Design review of the part built by this model. Coordinates are the model's own, in mm. A direction names the side the tool comes from. Coordinates: 2 decimals unless noted, no trailing zeros. Loops run counter-clockwise (first coordinate to the right, second up) from the corner with the lowest first, then second, coordinate; pieces in that order, holes last. Notation, with made-up numbers: (-17, 27) -> (36, 27) arc R12 cw to (36, 46) -> close; hole circle Ø10 at (-0.5, -10.5). An arc over 180 degrees is marked (long way). Answer in a Markdown table with one row per item.
```python
from build123d import *

# Parameters (mm, degrees)
SKETCH_1_R          = 7.25
SKETCH_1_R_2        = 4
EXTRUDE_1_DEPTH     = 6
SKETCH_2_R          = 3
SKETCH_2_R_2        = 1.5
CUT_EXTRUDE_1_DEPTH = 6


with BuildPart() as part:
    # 草图1 → 凸台-拉伸1 (new body)
    with BuildSketch(Plane.XY):
        with Locations((-10.375, 0)):
            Circle(SKETCH_1_R)
        with BuildLine():
            ThreePointArc((13.625, -4), (9.625, 0), (13.625, 4))
            Line((13.625, 4), (-4.328306689, 4))
            ThreePointArc((-4.328306689, 4), (-3.432341053, 2.088536987), (-3.125, 0))
            ThreePointArc((-3.125, 0), (-3.432341053, -2.088536987), (-4.328306689, -4))
            Line((-4.328306689, -4), (13.625, -4))
        make_face()
        with Locations((13.625, 0)):
            Circle(SKETCH_1_R_2)
    extrude(amount=EXTRUDE_1_DEPTH)

    # 草图2 → 切除-拉伸1 (cut)
    with BuildSketch(Plane.XY.offset(6)):
        with Locations((-10.375, 0)):
            Circle(SKETCH_2_R)
        with Locations((13.625, 0)):
            Circle(SKETCH_2_R_2)
    extrude(amount=-CUT_EXTRUDE_1_DEPTH, mode=Mode.SUBTRACT)


solid = part.part
```
(1) For pin 1 (2 mm diameter, centred on y = 4, z = 1, fed in from +X); pin 2 (6 mm diameter, centred on x = 5, y = 2, fed in from -Z); pin 3 (1 mm diameter, centred on x = -13, z = 3.5, fed in from +Y); pin 4 (2.5 mm diameter, centred on x = 13.625, y = 0, fed in from -Z), all flat-tipped, find the tip position at first contact; note any pin that passes through.
Evaluation:
| item | result |
|---|---|
| pin 1 | stops at x = 16.27 |
| pin 2 | stops at z = 0 |
| pin 3 | stops at y = 6.93 |
| pin 4 | passes through |
(2) Take a section at D-D on x = 2.5. Give the boundary of the cut face in (y, z).
Evaluation:
| item | result |
|---|---|
| outline | (-4, 0) -> (4, 0) -> (4, 6) -> (-4, 6) -> close |
(3) To check wall thickness, follow probe 1 along X at (y, z) = (-0.25, 2.2); probe 2 along Y at (x, z) = (-10.5, 0.7); probe 3 along Y at (x, z) = (-9.5, 5.45). State the ranges of each line that lie inside material, in increasing order.
Evaluation:
| item | result |
|---|---|
| probe 1 | x = -17.62 to -13.36, -7.39 to 12.15, 15.1 to 17.62 |
| probe 2 | y = -7.25 to -3, 3 to 7.25 |
| probe 3 | y = -7.2 to -2.87, 2.87 to 7.2 |
(4) Take a section at A-A on y = 0. Give the boundary of the cut face in (x, z) (3 decimals).
Evaluation:
| item | result |
|---|---|
| outline | (-17.625, 0) -> (-13.375, 0) -> (-13.375, 6) -> (-17.625, 6) -> close; (-7.375, 0) -> (12.125, 0) -> (12.125, 6) -> (-7.375, 6) -> close; (15.125, 0) -> (17.625, 0) -> (17.625, 6) -> (15.125, 6) -> close |
(5) Tool access review of faces 4 (the cylindrical face through (-17.62, 0.26, 2.96)), 5 (the flat face through (5, 4, 3)): name each direction out of +Z, -Z, +X, -X, +Y, -Y from which nothing blocks a thin tool from reaching the whole face with its end or side.
Evaluation:
| item | result |
|---|---|
| face 4 | +Z, -Z |
| face 5 | +Z, -Z, +X, +Y |
(6) Take a section at B-B on z = 1.5. Give the boundary of the cut face in (x, y) (3 decimals).
Evaluation:
| item | result |
|---|---|
| outline | (-4.328, -4) -> (13.625, -4) arc R4 ccw to (13.625, 4) -> (-4.328, 4) arc R7.25 ccw (long way) to start; hole circle Ø6 at (-10.375, 0); hole circle Ø3 at (13.625, 0) |
(7) Draft analysis for pull direction X (two halves, no side actions). For faces 1 (the flat face through (5, -4, 3)), 2 (the cylindrical face through (17.624, -0.088, 2.958)), 3 (the cylindrical face through (12.126, 0.066, 3.042)), state which applies: pulls with the +X half, pulls with the -X half, needs draft (parallel to the pull), parting line crosses it, or undercut.
Evaluation:
| item | result |
|---|---|
| face 1 | needs draft |
| face 2 | pulls with the +X half |
| face 3 | undercut |
(8) Take a section at C-C on x = -13. Give the boundary of the cut face in (y, z), and give its area (3 significant figures).
Evaluation:
| item | result |
|---|---|
| outline | (-6.76, 0) -> (-1.45, 0) -> (-1.45, 6) -> (-6.76, 6) -> close; (1.45, 0) -> (6.76, 0) -> (6.76, 6) -> (1.45, 6) -> close |
| area | 63.7 mm² |
